Autodesk Inventor part; units mm, degrees
ref_plane "YZ Plane" through (0, 0, 0) normal (1, 0, 0) x (0, 1, 0)
ref_plane "XZ Plane" through (0, 0, 0) normal (0, 1, 0) x (-1, 0, 0)
ref_plane "XY Plane" through (0, 0, 0) normal (0, 0, 1) x (1, 0, 0)
sketch "スケッチ1" plane through (0, 0, 0) normal (0, 0, 1) x (1, 0, 0)
  circle A0 centre (0, 0) radius 17.5
  line L0 (0, 0) -> (35, 0)
  line L1 (35, 0) -> (35, 20)
  line L2 (35, 20) -> (-1.2255, 17.457)
  line L3 (35, 20) -> (85, 20)
  line L4 (85, 20) -> (85, 0)
  line L5 (85, 0) -> (35, 0)
  line L6 (35, 0) -> (35, 20)
  line L7 (35, 0) -> (35, -20)
  line L8 (35, -20) -> (-1.2255, -17.457)
  line L9 (35, -20) -> (85, -20)
  line L10 (85, -20) -> (85, 0)
  point P0 (-1.2255, -17.457)
  dimension "d0" = 35
  dimension "d1" = 35
  dimension "d2" = 20
  dimension "d3" = 20
  dimension "d4" = 50
extrude "プレート1" add sketch "スケッチ1" along normal blind 2
sketch "スケッチ2" plane through (85, 22, -2) normal (0, 1, 0) x (-1, 0, 0)
  line L0 (50, 0) -> (0, 0)
  line L1 (0, 0) -> (0, -29.5)
  line L2 (0, -29.5) -> (50, -29.5)
  line L3 (50, -29.5) -> (50, 0)
edge flange "フランジ1" height 33.5 angle 90 thickness 2 bend radius 2 thickness toward (0, 1, 0) relief tear relief width 2 relief depth 1 corner gap 2 corner form 0 edges at (60, 20, 0) (60, -20, 0) wall of the first edge with corners at (35, 22, -2) (85, 22, -2) (85, 22, -31.5) (35, 22, -31.5)
bend "曲げ1"
corner "コーナー1"
sketch "スケッチ3" plane through (0, 0, 2) normal (0, 0, 1) x (1, 0, 0)
  circle A0 centre (0, 0) radius 13.5
  point P0 (0, 13.5)
  point P1 (-11.6913, 6.75)
  point P2 (-11.6913, -6.75)
  point P3 (0, -13.5)
  point P4 (11.6913, -6.75)
  point P5 (11.6913, 6.75)
  dimension "d16" = 27
  dimension "d19" = 360
hole "穴1" at (0, 13.5, 2) at (-11.6913, 6.75, 2) at (-11.6913, -6.75, 2) at (0, -13.5, 2) at (11.6913, -6.75, 2) at (11.6913, 6.75, 2) direction (0, 0, -1) diameter 3.2 end through all
sketch "スケッチ4" plane through (0, 0, 2) normal (0, 0, 1) x (1, 0, 0)
  arc A0 (-1.2255, 17.457) -> (-1.2255, -17.457) centre (0, 0) ccw
  circle A1 centre (0, 0) radius 6.25
  dimension "d28" = 12.5
extrude "押し出し1" cut sketch "スケッチ4" against normal blind 10
sketch "スケッチ5" plane through (35, 24, -31.5) normal (0, 1, 0) x (1, 0, 0)
  line L0 (0, 0) -> (0, -29.5)
  line L1 (0, -10) -> (50, -10)
  line L2 (50, -29.5) -> (50, 0)
  line L3 (50, 0) -> (0, 0)
  line L4 (10, 0) -> (10, -29.5)
  line L5 (0, -29.5) -> (50, -29.5)
  point P0 (-35, -31.5)
  point P1 (20, -10)
  point P2 (40, -10)
  dimension "d31" = 10
  dimension "d32" = 10
  dimension "d33" = 10
  dimension "d34" = 20
hole "穴2" at (55, 24, -21.5) at (75, 24, -21.5) direction (0, -1, 0) diameter 3.2 end through all
equation "\"d26\" = Thickness"
equation "\"d5\" = Thickness"
equation "\"d6\" = BendReliefWidth"
equation "\"d7\" = BendReliefDepth"
equation "\"d8\" = MinimumRemnant"
equation "\"d9\" = TransitionRadius"
equation "\"d12\" = BendRadius"
equation "\"d13\" = CornerReliefSize"
equation "\"d14\" = GapSize"
equation "\"d15\" = JacobiRadiusSize"
equation "\"BendRadius\" = Thickness"
equation "\"BendReliefWidth\" = Thickness"
equation "\"BendReliefDepth\" = 0.5 * Thickness"
equation "\"CornerReliefSize\" = 4 * Thickness"
equation "\"MinimumRemnant\" = 2 * Thickness"
equation "\"TransitionRadius\" = BendRadius"
equation "\"JacobiRadiusSize\" = BendRadius"
equation "\"GapSize\" = Thickness"
properties part number "servoplate1_forR0" material "アルミニウム 6061"
The listing builds one solid part. Answer for the finished solid, in the listing's coordinates (mm). A direction names the side the tool comes from. Coordinates: 2 decimals unless noted, no trailing zeros. Write each loop counter-clockwise with the first axis right and the second up, starting at its lowest first coordinate (ties: lowest second). Pieces come first, ordered by that corner, then holes. Notation, with made-up numbers: (-36.75, 82.5) - (-22.75, 82.5) arc R15 ccw to (-22.75, 108.5) - close; hole circle Ø7 at (67, 63). An arc over 180 degrees is marked (long way). Return JSON: item names as keys, results as strings. Group by question number.
Q1. The part is cut by section C-C on x = 55. Write down the section's boundary in (y, z), and give its area (3 significant figures).
Q2. Flat-ended cylindrical pins translate along their axes: pin 1 Ø1.2 at (y, z) = (23, -6.5) entering from -X; pin 2 Ø3 at (x, y) = (-6.5, 16.5) entering from -Z; pin 3 Ø5 at (x, z) = (55, -21.5) entering from +Y. Find the tip coordinate at first contact, or state that the pin passes through.
Q3. For a pull along X with two mould halves and no side action, classify faces 3 (the flat face through (44, 0, 0)), 4 (the cylindrical face through (-13.278, -6.542, 0.986)), 5 (the cylindrical face through (5.96, 1.88, 1.01)), 6 (the flat face through (17.141, -18.746, 0.986)) as +X half, -X half, draft (parallel to the pull), parting line (faces both ways), or undercut.
Q4. Which of the six approach directions +Z, -Z, +X, -X, +Y, -Y give full straight-line access (tool end or side, diameter ignored) to faces 1 (the cylindrical face through (-17.496, -0.368, 0.986)), 2 (the cylindrical face through (59.65, -21.43, -0.6))?
Q5. The part is cut by section A-A on z = -4. Write down the section's boundary in (x, y).
Q6. Find the intervals of material crossed by line 1 along Y through (x, z) = (68.5, -28.5); line 2 along X through (y, z) = (6.75, 0.8); line 3 along Y through (x, z) = (0, 1.45), in increasing order. Write a range as [from, to].
Q7. The part is cut by section D-D on x = 44. Write down the section's boundary in (y, z), and give its area (3 significant figures).
Q8. The part is cut by section B-B on y = 0. Write down the section's boundary in (x, z).
Evaluation:
{
 "1": {"outline": "(-24, -31.5) - (-22, -31.5) - (-22, -23.1) - (-24, -23.1) - close; (-24, -19.9) - (-22, -19.9) - (-22, -2) arc R2 cw to (-20, 0) - (20, 0) arc R2 cw to (22, -2) - (22, -19.9) - (24, -19.9) - (24, -2) arc R4 ccw to (20, 2) - (-20, 2) arc R4 ccw to (-24, -2) - close; (22, -31.5) - (24, -31.5) - (24, -23.1) - (22, -23.1) - close", "area": "204 mm2"},
 "2": {"pin 1": "stops at x = 35", "pin 2": "stops at z = 0", "pin 3": "stops at y = 24"},
 "3": {"face 3": "draft", "face 4": "undercut", "face 5": "undercut", "face 6": "-X half"},
 "4": {"face 1": "+Z, -Z, -X", "face 2": "-Z, +X, -X"},
 "5": {"outline": "(35, -24) - (85, -24) - (85, -22) - (35, -22) - close; (35, 22) - (85, 22) - (85, 24) - (35, 24) - close"},
 "6": {"line 1": "y = [-24, -22], [22, 24]", "line 2": "x = [-16.15, -13.29], [-10.09, 10.09], [13.29, 85]", "line 3": "y = [-17.54, -15.1], [-11.9, -6.25], [6.25, 11.9], [15.1, 17.54]"},
 "7": {"outline": "(-24, -31.5) - (-22, -31.5) - (-22, -2) arc R2 cw to (-20, 0) - (20, 0) arc R2 cw to (22, -2) - (22, -31.5) - (24, -31.5) - (24, -2) arc R4 ccw to (20, 2) - (-20, 2) arc R4 ccw to (-24, -2) - close", "area": "217 mm2"},
 "8": {"outline": "(-17.5, 0) - (-6.25, 0) - (-6.25, 2) - (-17.5, 2) - close; (6.25, 0) - (85, 0) - (85, 2) - (6.25, 2) - close"}
}
